Geometry: final body of the model. Coordinates: model frame, mm. Face numbers are marked on the shaded views. Give positions to 0.01 mm unless a question says otherwise; leave off trailing zeros. Loops run counter-clockwise (first coordinate to the right, second up) from the corner with the lowest first, then second, coordinate; pieces in that order, holes last. Notation, with made-up numbers: (60, 49.25) -> (66, 49.25) arc R9 cw to (66, 61.25) -> close; hole circle Ø1 at (61.5, -30). An arc over 180 degrees is marked (long way). Answer in a Markdown table with one row per item. Add a question column.
1) Line query: line 1 (Y direction, x = 0, z = 2.6); line 2 (Y direction, x = -15.5, z = 2.1) (3 decimals); line 3 (Y direction, x = 0.5, z = 3.4). Output: solid intervals per line, ascending. Write a range as from..to.
2) Section query A-A (y = 0). Return the cut outline in (x, z).
3) Section query D-D (z = 2.2). Give the number of separate pieces and of enclosed holes in the cut face, plus the area to 3 significant figures.
4) Draft query along X for the marked faces 1, 2 and 3. Return one class per face: +X half, -X half, draft (parallel to the pull), parting line (faces both ways), or undercut.
5) Section query C-C (y = 27). Return the cut outline in (x, z).
6) First-contact query: P1, Ø1.5, axis at x = 10.5, z = 3.5, coming from the +Y side; P2, Ø2, axis at y = -21, z = 1.5, coming from the -X side; P3, Ø2, axis at x = 15.5, z = 1, coming from the -Y side. Flat tips, straight axial feed; report the tip coordinate or a pass-through.
```python
from build123d import *

# Parameters (mm, degrees)
SKETCH25_R          = 30
SKETCH25_R_2        = 1.5
BOSS_EXTRUDE1_DEPTH = 5
SKETCH26_R          = 10
CUT_EXTRUDE1_DEPTH  = 5


with BuildPart() as part:
    # Sketch25 → Boss-Extrude1 (new body)
    with BuildSketch(Plane.XY):
        Circle(SKETCH25_R)
        with Locations((15.495, 15.495)):
            Circle(SKETCH25_R_2, mode=Mode.SUBTRACT)
        with Locations((-15.495, 15.495)):
            Circle(SKETCH25_R_2, mode=Mode.SUBTRACT)
        with Locations((-15.495, -15.495)):
            Circle(SKETCH25_R_2, mode=Mode.SUBTRACT)
        with Locations((15.495, -15.495)):
            Circle(SKETCH25_R_2, mode=Mode.SUBTRACT)
        with Locations((0, 27)):
            Circle(SKETCH25_R_2, mode=Mode.SUBTRACT)
        with Locations((27, 0)):
            Circle(SKETCH25_R_2, mode=Mode.SUBTRACT)
        with Locations((0, -27)):
            Circle(SKETCH25_R_2, mode=Mode.SUBTRACT)
        with Locations((-27, 0)):
            Circle(SKETCH25_R_2, mode=Mode.SUBTRACT)
    extrude(amount=BOSS_EXTRUDE1_DEPTH)

    # Sketch26 → Cut-Extrude1 (cut)
    with BuildSketch(Plane.XY.offset(5)):
        Circle(SKETCH26_R)
        with Locations((-130.084851818, -8.286873835)):
            Circle(SKETCH26_R)
    extrude(amount=-CUT_EXTRUDE1_DEPTH, mode=Mode.SUBTRACT)


solid = part.part
```
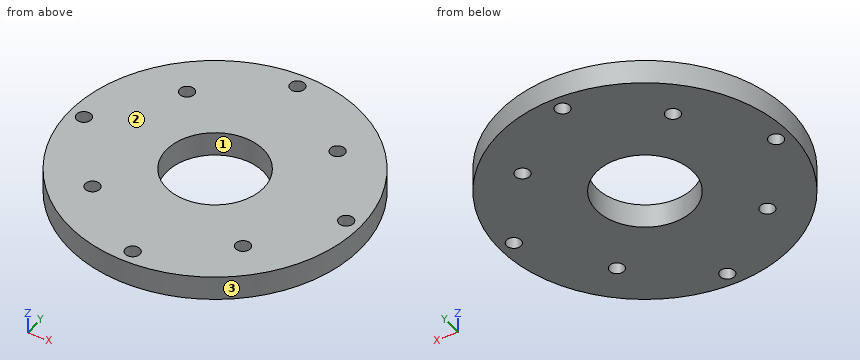
Evaluation:
| question | item | result |
|---|---|---|
| 1 | line 1 | -30..-28.5, -25.5..-10, 10..25.5, 28.5..30 |
| 1 | line 2 | -25.686..-16.995, -13.995..13.995, 16.995..25.686 |
| 1 | line 3 | -30..-28.41, -25.59..-9.99, 9.99..25.59, 28.41..30 |
| 2 | outline | (-30, 0) -> (-28.5, 0) -> (-28.5, 5) -> (-30, 5) -> close; (-25.5, 0) -> (-10, 0) -> (-10, 5) -> (-25.5, 5) -> close; (10, 0) -> (25.5, 0) -> (25.5, 5) -> (10, 5) -> close; (28.5, 0) -> (30, 0) -> (30, 5) -> (28.5, 5) -> close |
| 3 | separate pieces | 1 |
| 3 | enclosed holes | 9 |
| 3 | area | 2,460 mm² |
| 4 | face 1 | undercut |
| 4 | face 2 | draft |
| 4 | face 3 | parting line |
| 5 | outline | (-13.08, 0) -> (-1.5, 0) -> (-1.5, 5) -> (-13.08, 5) -> close; (1.5, 0) -> (13.08, 0) -> (13.08, 5) -> (1.5, 5) -> close |
| 6 | P1 | y = 28.37 |
| 6 | P2 | x = -22.36 |
| 6 | P3 | y = -26.26 |
